Read the model definition and answer for the solid it produces. Units are mm, in the model's axes. A direction names the side the tool comes from. Coordinates: 2 decimals unless noted, no trailing zeros. Loops run counter-clockwise (first coordinate to the right, second up) from the corner with the lowest first, then second, coordinate; pieces in that order, holes last.
from build123d import *

# Parameters (mm, degrees)
F2_R = 1.26999


# Not quite as in the source:
# - a fillet or chamfer is up to 0.001 mm smaller than in the source, because OpenCascade refuses the exact size


with BuildPart() as f1:
    # F0 (on Front) → F1 (revolve)
    with BuildSketch(Plane.XZ):
        with BuildLine():
            Line((76.2, 12.7), (76.2, 279.4))
            ThreePointArc((76.2, 279.4), (74.0202749456, 294.1210347534), (67.6681549524, 307.5787699682))
            Line((67.6681549524, 307.5787699682), (55.0659225238, 326.4821186111))
            ThreePointArc((55.0659225238, 326.4821186111), (51.8898625272, 333.2109862185), (50.8, 340.5715035952))
            Line((50.8, 340.5715035952), (50.8, 381))
            Line((50.8, 381), (48.26, 381))
            Line((48.26, 381), (48.26, 340.5715035952))
            ThreePointArc((48.26, 340.5715035952), (49.4588487799, 332.4749344808), (52.9525147762, 325.0731801126))
            Line((52.9525147762, 325.0731801126), (65.5547472047, 306.1698314698))
            ThreePointArc((65.5547472047, 306.1698314698), (71.5892611984, 293.3849830157), (73.66, 279.4))
            Line((73.66, 279.4), (73.66, 12.7))
            ThreePointArc((73.66, 12.7), (70.6842048969, 5.5157951031), (63.5, 2.54))
            Line((63.5, 2.54), (0, 2.54))
            Line((0, 2.54), (0, 0))
            Line((0, 0), (63.5, 0))
            ThreePointArc((63.5, 0), (72.4802561211, 3.7197438789), (76.2, 12.7))
        make_face()
    revolve(axis=Axis((0, 0, 199.2018222809), (0, 0, 1)))

    # F2 (radius 1.27 in the source; OpenCascade refuses exactly that, so slightly less here)
    f2_edges = [f1.edges().sort_by_distance(p)[0] for p in [
        (-50.8, 0, 381),
        (-48.26, 0, 381),
    ]]
    fillet(f2_edges, radius=F2_R)


solid = f1.part
Q1. A cutting plane is placed at B-B (z = 30). Give the vertices of the cut face in (x, y), then the cut area to 3 significant figures.
Findings below:
outline: circle Ø152.4 at (0, 0); hole circle Ø147.32 at (0, 0)
area: 1,200 mm2
Q2. Which of the six approach directions +Z, -Z, +X, -X, +Y, -Y give full straight-line access (tool end or side, diameter ignored) to faces 1 (the face through (-11.65, -52.463, 323.891)), 2 (the face through (-60.47, -46.367, 147.917)), 3 (the face through (-11.012, -49.592, 360.425))?
Findings below:
face 1: none
face 2: +Z, -Z
face 3: +Z
Q3. Determine the mould class of faces 4 (the face through (46.03, 14.5, 359.88)), 5 (the face through (1, 1, 0)), 6 (the face through (-44.184, -33.879, 325.564)) for opening direction X: +X half, -X half, draft (parallel to the pull), parting line (faces both ways), or undercut.
Findings below:
face 4: undercut
face 5: draft
face 6: parting line
Q4. Straight lines are drawn through the part: probe 1 along Y at (x, z) = (0, 150.5); probe 2 along Y at (x, z) = (-1, 348); probe 3 along X at (y, z) = (1, 243). For each, find the intervals that lie inside material, in ascending order.
Findings below:
probe 1: y = -76.2 to -73.66, 73.66 to 76.2
probe 2: y = -50.79 to -48.25, 48.25 to 50.79
probe 3: x = -76.19 to -73.65, 73.65 to 76.19
Q5. Flat-ended cylindrical pins translate along their axes: pin 1 Ø6 at (x, z) = (27, 280.5) entering from -Y; pin 2 Ø6 at (y, z) = (44, 319.5) entering from -X; pin 3 Ø1.5 at (x, z) = (25, 296.5) entering from +Y. Find the tip coordinate at first contact, or state that the pin passes through.
Findings below:
pin 1: stops at y = -72.31
pin 2: stops at x = -44.54
pin 3: stops at y = 69.22
Q6. A cutting plane is placed at A-A (z = 355). Give the vertices of the cut face in (x, y).
Findings below:
outline: circle Ø101.6 at (0, 0); hole circle Ø96.52 at (0, 0)
